Check sheet for the modelled part. Datum: model origin and axes. Units: mm. A direction names the side the tool comes from. Coordinates: 2 decimals unless noted, no trailing zeros. Order: outer loops, then holes, each group sorted by start corner. A loop starts at its lowest first (then second) coordinate and runs counter-clockwise, first axis right, second up.
from build123d import *

# Parameters (mm, degrees)
EXTRUDE_DEPTH = 3.3
SKETCH001_R   = 1.5
POCKET_DEPTH  = 3.301
PAD_DEPTH     = 2
FILLET_R      = 1
FILLET001_R   = 1
FILLET002_R   = 1


with BuildPart() as part:
    # Sketch → Extrude (new body)
    with BuildSketch(Plane.XY):
        with BuildLine():
            ThreePointArc((3.5, 21.5), (0, 25), (-3.5, 21.5))
            Line((-3.5, 21.5), (-3.5, 19.691369))
            ThreePointArc((-3.5, 19.691369), (0, -20), (3.5, 19.691369))
            Line((3.5, 19.691369), (3.5, 21.5))
        make_face()
    extrude(amount=EXTRUDE_DEPTH)

    # Sketch001 → Pocket (cut, through all)
    with BuildSketch(Plane.XY.offset(3.3)):
        with Locations((0, 21.5)):
            Circle(SKETCH001_R)
    extrude(amount=-POCKET_DEPTH, mode=Mode.SUBTRACT)

    # Sketch002 → Pad (new body)
    with BuildSketch(Plane.XY.offset(3.3)):
        with BuildLine():
            Line((-1.5, 13.5), (-1.5, -5))
            ThreePointArc((-1.5, -5), (0, -6.5), (1.5, -5))
            Line((1.5, 13.5), (1.5, -5))
            ThreePointArc((1.5, 13.5), (0, 15.000005), (-1.5, 13.5))
        make_face()
        with BuildLine():
            ThreePointArc((-3.2, 8.565466), (0, -9.143698), (3.2, 8.565466))
            Line((3.2, 11.565466), (3.2, 8.565466))
            ThreePointArc((-3.2, 11.565466), (0, -12), (3.2, 11.565466))
            Line((-3.2, 11.565466), (-3.2, 8.565466))
        make_face()
    extrude(amount=PAD_DEPTH)

    # Fillet
    fillet_edges = [part.edges().sort_by_distance(p)[0] for p in [
        (0, -12, 5.3),
    ]]
    fillet(fillet_edges, radius=FILLET_R)

    # Fillet001
    fillet001_edges = [part.edges().sort_by_distance(p)[0] for p in [
        (0, -9.143698, 5.3),
    ]]
    fillet(fillet001_edges, radius=FILLET001_R)

    # Fillet002
    fillet002_edges = [part.edges().sort_by_distance(p)[0] for p in [
        (1.5, 4.25, 5.3),
    ]]
    fillet(fillet002_edges, radius=FILLET002_R)


solid = part.part
(1) Cross-section at B-B (z = 0.5). Enter the section's corners in (x, y), and give its area (3 significant figures).
Filled in:
outline: (-3.5, 19.69) arc R20 ccw (long way) to (3.5, 19.69) - (3.5, 21.5) arc R3.5 ccw to (-3.5, 21.5) - close; hole circle Ø3 at (0, 21.5)
area: 1,280 mm2
(2) Thickness scan on probe 1 along X at (y, z) = (0, 3.5); probe 2 along Y at (x, z) = (0, 2.4); probe 3 along X at (y, z) = (1.5, 4.95). Record the ranges inside material, lowest first.
Filled in:
probe 1: x = -12 to -9.14, -1.5 to 1.5, 9.14 to 12
probe 2: y = -20 to 20, 23 to 25
probe 3: x = -11.66 to -9.26, -1.26 to 1.26, 9.26 to 11.66
(3) Release check for a two-part mould opening along X. For faces 6 (the flat face through (3.5, 21, 2)), 7 (the cylindrical face through (0, 25, 2)), 8 (the cylindrical face through (1.215, 4.12, 4.999)), 9 (the flat face through (4, -2, 3.3)) record: +X half, -X half, draft (parallel to the pull), parting line (faces both ways), or undercut.
Filled in:
face 6: +X half
face 7: parting line
face 8: undercut
face 9: undercut
(4) Cross-section at C-C (y = 13). Enter the section's corners in (x, z).
Filled in:
outline: (-15.2, 0) - (15.2, 0) - (15.2, 3.3) - (1.5, 3.3) - (1.5, 4.3) arc R1 ccw to (0.5, 5.3) - (-0.5, 5.3) arc R1 ccw to (-1.5, 4.3) - (-1.5, 3.3) - (-15.2, 3.3) - close
(5) Tool access check on faces 1 (the cylindrical face through (-0.83, -19.983, 1.627)), 2 (the flat face through (0, -2, 0)), 3 (the cylindrical face through (0, -12, 4)), 4 (the flat face through (-3.2, 10, 4)), 5 (the flat face through (-3.5, 21, 2)). Record the directions out of +Z, -Z, +X, -X, +Y, -Y that give a thin tool (end or side, any length) a straight path to the whole face; none if there is none.
Filled in:
face 1: +Z, -Z
face 2: -Z, +X, -X, +Y, -Y
face 3: +Z
face 4: +Z, +Y
face 5: +Z, -Z, -X, +Y
(6) Go/stop test with flat-tipped pins: P1, Ø1.4, axis at y = 20.5, z = 2, coming from the -X side; P2, Ø1.6, axis at y = 10, z = 4.5, coming from the -X side; P3, Ø1.5, axis at x = 1.5, z = 2.5, coming from the +Y side; P4, Ø1.8, axis at x = 0, y = 21.5, coming from the +Z side. Record where each tip stops, or that it passes through.
Filled in:
P1: stops at x = -3.5
P2: stops at x = -7.69
P3: stops at y = 24.92
P4: passes through
(7) Cross-section at A-A (y = 20.5). Enter the section's corners in (x, z), and give its area (3 significant figures).
Filled in:
outline: (-3.5, 0) - (-1.12, 0) - (-1.12, 3.3) - (-3.5, 3.3) - close; (1.12, 0) - (3.5, 0) - (3.5, 3.3) - (1.12, 3.3) - close
area: 15.7 mm2
(8) Cross-section at D-D (x = 13.5). Enter the section's corners in (y, z), and give its area (3 significant figures).
Filled in:
outline: (-14.76, 0) - (14.76, 0) - (14.76, 3.3) - (-14.76, 3.3) - close
area: 97.4 mm2
